from build123d import *

# Parameters (mm, degrees)
BOSS_EXTRUDE1_DEPTH = 25
SKETCH2_R           = 5
BOSS_EXTRUDE2_DEPTH = 1.7
SKETCH3_R           = 1
BOSS_EXTRUDE3_DEPTH = 10


with BuildPart() as part:
    # Sketch1 → Boss-Extrude1 (new body)
    with BuildSketch(Plane.XY):
        with BuildLine():
            Line((-6.633249581, -7.55), (6.633249581, -7.55))
            ThreePointArc((6.633249581, -7.55), (10.05, 0), (6.633249581, 7.55))
            Line((6.633249581, 7.55), (-6.633249581, 7.55))
            ThreePointArc((-6.633249581, 7.55), (-10.05, 0), (-6.633249581, -7.55))
        make_face()
    extrude(amount=BOSS_EXTRUDE1_DEPTH)

    # Sketch2 → Boss-Extrude2 (add)
    with BuildSketch(Plane.XY.offset(25)):
        Circle(SKETCH2_R)
    extrude(amount=BOSS_EXTRUDE2_DEPTH)

    # Sketch3 → Boss-Extrude3 (add)
    with BuildSketch(Plane.XY.offset(26.7)):
        Circle(SKETCH3_R)
    extrude(amount=BOSS_EXTRUDE3_DEPTH)


solid = part.part
Verification items for the finished model (mm, model axes). A direction names the side the tool comes from. Round coordinates to 2 decimals unless told otherwise and drop trailing zeros. Loops run counter-clockwise (first coordinate to the right, second up) from the corner with the lowest first, then second, coordinate; pieces in that order, holes last. Notation, with made-up numbers: (42, 11) - (56, 11) arc R9 ccw to (56, 23) - close; hole circle Ø2 at (14, 74.5). An arc over 180 degrees is marked (long way). Use a Markdown table: item, result. Add a question column.
1. Section check D-D, the plane y = 2.75. Record the boundary of the cut face in (x, z), plus the area to 3 significant figures.
2. Section check C-C, the plane z = 21.5. Record the boundary of the cut face in (x, y), plus the area to 3 significant figures.
3. Section check B-B, the plane x = 0. Record the boundary of the cut face in (y, z).
4. Section check A-A, the plane y = 0. Record the boundary of the cut face in (x, z).
5. Thickness scan on probe 1 along Z at (x, y) = (-1.5, 0.5); probe 2 along Z at (x, y) = (-5.5, -0.5); probe 3 along Y at (x, z) = (7, 15.5). Record the ranges inside material, lowest first. Write a range as [from, to].
6. Access from +Z, -Z, +X, -X, +Y, -Y to the whole of each face (thin tool, end or side, straight path). Record for faces 1 (the face through (-2, 5, 25)), 2 (the face through (0, 0, 36.7)).
7. Gauge pin test, flat ends, axial feed: pin 1 (4 mm diameter, centred on x = 3.5, y = -0.5, fed in from +Z); pin 2 (1.5 mm diameter, centred on y = 3, z = 32, fed in from -X). Record the tip position at first contact, or that the pin passes through.
Checks:
| question | item | result |
|---|---|---|
| 1 | outline | (-9.67, 0) - (9.67, 0) - (9.67, 25) - (4.18, 25) - (4.18, 26.7) - (-4.18, 26.7) - (-4.18, 25) - (-9.67, 25) - close |
| 1 | area | 498 mm^2 |
| 2 | outline | (-6.63, -7.55) - (6.63, -7.55) arc R10.05 ccw to (6.63, 7.55) - (-6.63, 7.55) arc R10.05 ccw to start |
| 2 | area | 272 mm^2 |
| 3 | outline | (-7.55, 0) - (7.55, 0) - (7.55, 25) - (5, 25) - (5, 26.7) - (1, 26.7) - (1, 36.7) - (-1, 36.7) - (-1, 26.7) - (-5, 26.7) - (-5, 25) - (-7.55, 25) - close |
| 4 | outline | (-10.05, 0) - (10.05, 0) - (10.05, 25) - (5, 25) - (5, 26.7) - (1, 26.7) - (1, 36.7) - (-1, 36.7) - (-1, 26.7) - (-5, 26.7) - (-5, 25) - (-10.05, 25) - close |
| 5 | probe 1 | z = [0, 26.7] |
| 5 | probe 2 | z = [0, 25] |
| 5 | probe 3 | y = [-7.21, 7.21] |
| 6 | face 1 | +Z |
| 6 | face 2 | +Z, +X, -X, +Y, -Y |
| 7 | pin 1 | stops at z = 26.7 |
| 7 | pin 2 | passes through |
